Verification items for the finished model (mm, model axes). A direction names the side the tool comes from. Coordinates: 2 decimals unless noted, no trailing zeros. Write each loop counter-clockwise with the first axis right and the second up, starting at its lowest first coordinate (ties: lowest second). Pieces come first, ordered by that corner, then holes. Notation, with made-up numbers: (6.25, 55.5) - (40.25, 55.5) arc R13 cw to (40.25, 70.5) - close; hole circle Ø3 at (-3.75, -27.5). An arc over 180 degrees is marked (long way). Use one line per item in the form item = value. Start each with the question number.
(1) Sectioned sample at C-C (x = 19). Record the cut outline in (y, z).
(2) Sectioned sample at D-D (y = -3). Record the cut outline in (x, z), and give its area (3 significant figures).
(3) Material ranges on line 1 (Z direction, x = 21, y = -5.5); line 2 (X direction, y = -4.5, z = 12); line 3 (X direction, y = -2.25, z = 71.5), recorded low to high. Write a range as [from, to].
(4) Sectioned sample at A-A (y = 2). Record the cut outline in (x, z).
(5) Sectioned sample at B-B (z = 63.5). Record the cut outline in (x, y).
(6) Mould release check, pull along X, two halves, no side actions. Record for faces 1 (the flat face through (18, -1, 79)), 2 (the cylindrical face through (11.641, -8.524, 0.74)), 3 (the flat face through (-10.5, 0, 39)), 4 (the flat face through (28.17, 0.88, 38.97)): released by +X, released by -X, zero draft, split by the parting line, or undercut.
(7) Gauge pin test, flat ends, axial feed: pin 1 Ø1 at (x, z) = (36.5, 67) entering from -Y; pin 2 Ø1 at (y, z) = (2.5, 53.5) entering from +X; pin 3 Ø8 at (x, y) = (2, -5.5) entering from -Z; pin 4 Ø1.2 at (x, z) = (30.5, 1) entering from -Y. Record the tip position at first contact, or that the pin passes through.
(8) Tool access check on faces 5 (the flat face through (18, -1, 0)), 6 (the flat face through (10.5, -2, 39)), 7 (the flat face through (-9, 0, 39)). Record the directions out of +Z, -Z, +X, -X, +Y, -Y that give a thin tool (end or side, any length) a straight path to the whole face; none if there is none.
from build123d import *

# Parameters (mm, degrees)
F1_DEPTH = 79
F4_DEPTH = 1.5
F5_DEPTH = 1.5


with BuildPart() as f1:
    # F0 (on Top) → F1 (new body)
    with BuildSketch(Plane.XY):
        Polygon((-9, -9), (-9, 9), (9, 9), (9, -9), (8.7474873289, -10.5), (9.1674439609, -11.7616653442), (10.5, -11.7616653442), (10.5, -11.3207034852), (10.5, 8.8543308896), (46.3423287091, -7.3207034852), (46.9593341512, -5.9534784545), (10.5, 10.5), (-10.5, 10.5), (-10.5, -11.7616653442), (-9.1674439609, -11.7616653442), (-8.7474873289, -10.5), align=None)
    extrude(amount=F1_DEPTH)

    # F3 (on offset) → F4 (join)
    with BuildSketch(Plane.XY.offset(79)):
        with BuildLine():
            Line((-9, -9), (-9, 9))
            Line((-9, 9), (9, 9))
            Line((9, 9), (9, -9))
            Line((9, -9), (8.7474873289, -10.5))
            Line((8.7474873289, -10.5), (9.1674439609, -11.7616653442))
            Line((9.1674439609, -11.7616653442), (10.5, -11.7616653442))
            Line((10.5, -11.7616653442), (10.5, -11.3207034852))
            ThreePointArc((10.5, -11.3207034852), (11.6715728753, -8.4922763604), (14.5, -7.3207034852))
            Line((14.5, -7.3207034852), (46.3423287091, -7.3207034852))
            Line((46.3423287091, -7.3207034852), (46.9593341512, -5.9534784545))
            Line((46.9593341512, -5.9534784545), (10.5, 10.5))
            Line((10.5, 10.5), (-10.5, 10.5))
            Line((-10.5, 10.5), (-10.5, -11.7616653442))
            Line((-10.5, -11.7616653442), (-9.1674439609, -11.7616653442))
            Line((-9.1674439609, -11.7616653442), (-8.7474873289, -10.5))
            Line((-8.7474873289, -10.5), (-9, -9))
        make_face()
    extrude(amount=-F4_DEPTH)

    # F0 (on Top) → F5 (join)
    with BuildSketch(Plane.XY):
        with BuildLine():
            Line((10.5, 8.8543308896), (10.5, -11.3207034852))
            ThreePointArc((10.5, -11.3207034852), (11.6715728753, -8.4922763604), (14.5, -7.3207034852))
            Line((14.5, -7.3207034852), (46.3423287091, -7.3207034852))
            Line((46.3423287091, -7.3207034852), (10.5, 8.8543308896))
        make_face()
    extrude(amount=F5_DEPTH)


solid = f1.part
Answers below:
q1.outline = (-7.32, 0) - (6.66, 0) - (6.66, 79) - (-7.32, 79) - (-7.32, 77.5) - (5.02, 77.5) - (5.02, 1.5) - (-7.32, 1.5) - close
q2.outline = (-10.5, 0) - (-9, 0) - (-9, 79) - (-10.5, 79) - close; (9, 0) - (40.41, 0) - (40.41, 79) - (9, 79) - close; hole (10.5, 1.5) - (36.77, 1.5) - (36.77, 77.5) - (10.5, 77.5) - close
q2.area = 604 mm2
q3.line_1 = [0, 1.5], [77.5, 79]
q3.line_2 = [-10.5, -9], [9, 10.5], [40.09, 43.74]
q3.line_3 = [-10.5, -9], [9, 10.5], [35.11, 38.75]
q4.outline = (-10.5, 0) - (-9, 0) - (-9, 79) - (-10.5, 79) - close; (9, 0) - (29.34, 0) - (29.34, 79) - (9, 79) - close; hole (10.5, 1.5) - (25.69, 1.5) - (25.69, 77.5) - (10.5, 77.5) - close
q5.outline = (-10.5, -11.76) - (-9.17, -11.76) - (-8.75, -10.5) - (-9, -9) - (-9, 9) - (9, 9) - (9, -9) - (8.75, -10.5) - (9.17, -11.76) - (10.5, -11.76) - (10.5, 8.85) - (46.34, -7.32) - (46.96, -5.95) - (10.5, 10.5) - (-10.5, 10.5) - close
q6.face_1 = zero draft
q6.face_2 = released by +X
q6.face_3 = released by -X
q6.face_4 = undercut
q7.pin_1 = -3.1
q7.pin_2 = 29.34
q7.pin_3 = through
q7.pin_4 = -7.32
q8.face_5 = -Z, +X, -X, +Y, -Y
q8.face_6 = -Y
q8.face_7 = +Z, -Z
